Part print with two shaded views. Sizes in mm from the minimum x, y, z corner. A direction names the side the tool comes from. Round coordinates to 2 decimals unless told otherwise and drop trailing zeros. Loops run counter-clockwise (first coordinate to the right, second up) from the corner with the lowest first, then second, coordinate; pieces in that order, holes last.
(1) Flat gauge pins, fed straight in: pin 1 (15 mm diameter, centred on x = 32.5, y = 46, fed in from +Z); pin 2 (6 mm diameter, centred on y = 34, z = 54, fed in from -X); pin 3 (5 mm diameter, centred on x = 58, y = 39.5, fed in from +Z). Where does each tip first touch, or does it go through?
(2) Cut at B-B on y = 27. List the corners of the cut face in (x, z).
(3) Cut at C-C on x = 33. List the corners of the cut face in (y, z).
(4) Tool access for the marked faces 1 and 2: list every direction of +Z, -Z, +X, -X, +Y, -Y with a clear straight run to the whole face (end or side of a thin tool).
(5) Cut at D-D on y = 58. List the corners of the cut face in (x, z), then the cut area to 3 significant figures.
(6) Cut at A-A on z = 65. List the corners of the cut face in (x, y) (1 decimal), then the cut area to 3 significant figures.
(7) Mould opens along X. For the marked faces 3, 4, 5 and 6 say: +X half, -X half, draft (parallel to the pull), parting line (faces both ways), or undercut.
(8) Probe probe 1 along X at (y, z) = (32, 13); probe 2 along X at (y, z) = (32.5, 153.5); probe 3 along Z at (x, y) = (55, 17). List the from-to ranges inside material, lowest first.
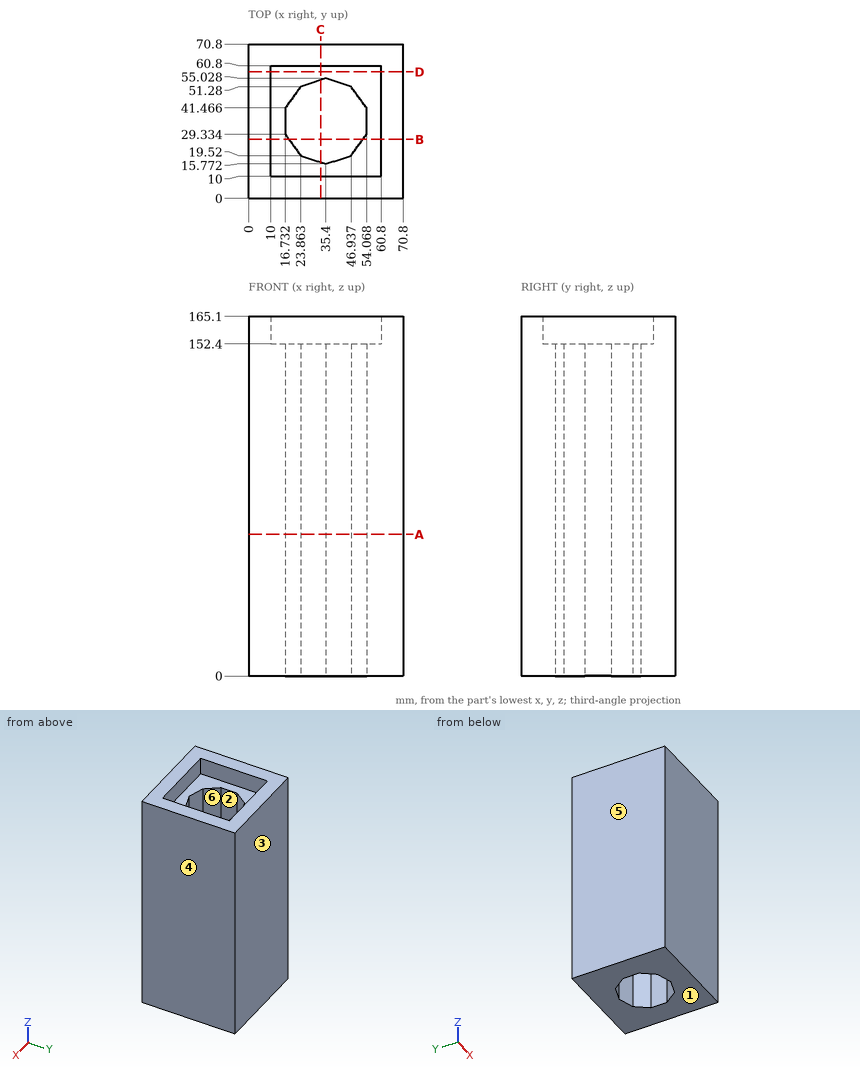
Final values:
1. pin 1: passes through
1. pin 2: stops at x = 0
1. pin 3: stops at z = 152.4
2. outline: (0, 0) - (18.43, 0) - (18.43, 152.4) - (10, 152.4) - (10, 165.1) - (0, 165.1) - close; (52.37, 0) - (70.8, 0) - (70.8, 165.1) - (60.8, 165.1) - (60.8, 152.4) - (52.37, 152.4) - close
3. outline: (0, 0) - (16.55, 0) - (16.55, 152.4) - (10, 152.4) - (10, 165.1) - (0, 165.1) - close; (54.25, 0) - (70.8, 0) - (70.8, 165.1) - (60.8, 165.1) - (60.8, 152.4) - (54.25, 152.4) - close
4. face 1: -Z, +X, -X, +Y, -Y
4. face 2: +Z, -Z
5. outline: (0, 0) - (70.8, 0) - (70.8, 165.1) - (60.8, 165.1) - (60.8, 152.4) - (10, 152.4) - (10, 165.1) - (0, 165.1) - close
5. area: 11,000 mm2
6. outline: (0, 0) - (70.8, 0) - (70.8, 70.8) - (0, 70.8) - close; hole (16.7, 29.3) - (23.9, 19.5) - (35.4, 15.8) - (46.9, 19.5) - (54.1, 29.3) - (54.1, 41.5) - (46.9, 51.3) - (35.4, 55) - (23.9, 51.3) - (16.7, 41.5) - close
6. area: 3,880 mm2
7. face 3: draft
7. face 4: +X half
7. face 5: -X half
7. face 6: undercut
8. probe 1: x = 0 to 16.73, 54.07 to 70.8
8. probe 2: x = 0 to 10, 60.8 to 70.8
8. probe 3: z = 0 to 152.4
